Read the model definition and answer for the solid it produces. Units are mm, in the model's axes. A direction names the side the tool comes from. Round coordinates to 2 decimals unless told otherwise and drop trailing zeros. Order: outer loops, then holes, each group sorted by start corner. A loop starts at its lowest first (then second) coordinate and runs counter-clockwise, first axis right, second up. Notation, with made-up numbers: (39, 42.5) - (47, 42.5) arc R14 cw to (47, 53.5) - close; hole circle Ø7 at (32, 46). An arc over 180 degrees is marked (long way). Put each result on its own line as item: value. Start each with the question number.
Q1. Section A-A on x = 0 is taken. Give the vertices of the cut face in (y, z).
Q2. Find the intervals of material crossed by line 1 along X through (y, z) = (6, 0); line 2 along Z through (x, y) = (0, 3); line 3 along Z through (x, y) = (113.5, 9.5), in increasing order. Write a range as from..to.
Q3. Section B-B on y = 13.5 is taken. Give the vertices of the cut face in (x, z), then the cut area to 3 significant figures.
Q4. For a pull along Z with two mould halves and no side action, classify faces 1 (the face through (188.4, 4.9, 54.8)), 2 (the face through (-113.35, 5.07, -64.18)), 3 (the face through (111.43, 5.07, -66.42)) as pulls with the +Z half, pulls with the -Z half, needs draft (parallel to the pull), parting line crosses it, or undercut.
Q5. Which of the six approach directions +Z, -Z, +X, -X, +Y, -Y give full straight-line access (tool end or side, diameter ignored) to faces 4 (the face through (69, 10, -3)), 5 (the face through (-80, 15, 0)), 6 (the face through (-133.6, 4.9, -111.4))?
Q6. Section D-D on x = 65 is taken. Give the vertices of the cut face in (y, z), then the cut area to 3 significant figures.
Q7. Each of these flat-tipped pins is pushed along its axis until it touches: pin 1 Ø5 at (x, y) = (163, 7.5) entering from +Z; pin 2 Ø8 at (y, z) = (6.5, 102) entering from +X; pin 3 Ø5 at (x, y) = (155, 7.5) entering from -Z. Where does it stop, or does it pass through?
Q8. Section C-C on z = -107.5 is taken. Give the vertices of the cut face in (x, y).
from build123d import *

# Parameters (mm, degrees)
SKETCH2_R           = 120
SKETCH2_R_2         = 60
BOSS_EXTRUDE1_DEPTH = 10
BOSS_EXTRUDE2_DEPTH = 10
CIRPATTERN1_COUNT   = 3
FILLET1_R           = 80
BOSS_EXTRUDE3_DEPTH = 10


with BuildPart() as part:
    # Sketch2 → Boss-Extrude1 (new body)
    with BuildSketch(Plane(origin=(0, 0, 0), x_dir=(1, 0, 0), z_dir=(0, 1, 0))):
        with Locations(Location((0, 0, 0), (0, 0, 270))):
            Circle(SKETCH2_R)
        with Locations(Location((0, 0, 0), (0, 0, 270))):
            Circle(SKETCH2_R_2, mode=Mode.SUBTRACT)
    extrude(amount=BOSS_EXTRUDE1_DEPTH)

    # Sketch2_3 → Boss-Extrude2 (add)
    with BuildSketch(Plane(origin=(0, 0, 0), x_dir=(1, 0, 0), z_dir=(0, 1, 0))):
        with BuildLine():
            Line((183.198176877, 60), (103.923048454, 60))
            ThreePointArc((103.923048454, 60), (115.911099155, 31.058285412), (120, 0))
            ThreePointArc((120, 0), (115.911099155, -31.058285412), (103.923048454, -60))
            Line((103.923048454, -60), (183.198176877, -60))
            Line((183.198176877, -60), (193.804778595, -49.393398282))
            ThreePointArc((193.804778595, -49.393398282), (200, 0), (193.804778595, 49.393398282))
            Line((193.804778595, 49.393398282), (183.198176877, 60))
        make_face()
    boss_extrude2 = extrude(amount=BOSS_EXTRUDE2_DEPTH)

    # CirPattern1: Boss-Extrude2 ×3 about axis
    cirpattern1_axis = Axis((0, 0, 0), (0, 1, 0))
    for i in range(1, CIRPATTERN1_COUNT):
        add(boss_extrude2.rotate(cirpattern1_axis, i * 360 / CIRPATTERN1_COUNT))

    # Fillet1
    fillet1_edges = [part.edges().sort_by_distance(p)[0] for p in [
        (103.923048454, 5, -60),
        (103.923048454, 5, 60),
        (-103.923048454, 5, -60),
        (0, 5, -120),
        (0, 5, 120),
        (-103.923048454, 5, 60),
    ]]
    fillet(fillet1_edges, radius=FILLET1_R)

    # Sketch3 → Boss-Extrude3 (add)
    with BuildSketch(Plane(origin=(0, 10, 0), x_dir=(1, 0, 0), z_dir=(0, 1, 0))):
        with BuildLine():
            Line((-5.773502692, 10), (-8.660254038, 5))
            ThreePointArc((-8.660254038, 5), (-5, 8.660254038), (0, 10))
            Line((0, 10), (-5.773502692, 10))
        make_face()
        with BuildLine():
            ThreePointArc((8.660254038, 5), (10, 0), (8.660254038, -5))
            Line((8.660254038, -5), (11.547005384, 0))
            Line((11.547005384, 0), (8.660254038, 5))
        make_face()
        with BuildLine():
            Line((-5.773502692, -10), (0, -10))
            ThreePointArc((0, -10), (-5, -8.660254038), (-8.660254038, -5))
            Line((-8.660254038, -5), (-5.773502692, -10))
        make_face()
        with BuildLine():
            ThreePointArc((-8.660254038, -5), (-5, -8.660254038), (0, -10))
            ThreePointArc((0, -10), (5, -8.660254038), (8.660254038, -5))
            ThreePointArc((8.660254038, -5), (10, 0), (8.660254038, 5))
            ThreePointArc((8.660254038, 5), (5, 8.660254038), (0, 10))
            ThreePointArc((0, 10), (-5, 8.660254038), (-8.660254038, 5))
            ThreePointArc((-8.660254038, 5), (-10, 0), (-8.660254038, -5))
        make_face()
        with BuildLine():
            Line((8.660254038, 5), (11.547005384, 0))
            Line((11.547005384, 0), (22.802389662, 19.494897428))
            ThreePointArc((22.802389662, 19.494897428), (15, 25.980762114), (5.481881586, 29.494897428))
            Line((5.481881586, 29.494897428), (-5.773502692, 10))
            Line((-5.773502692, 10), (0, 10))
            ThreePointArc((0, 10), (5, 8.660254038), (8.660254038, 5))
        make_face()
        with BuildLine():
            ThreePointArc((8.660254038, -5), (5, -8.660254038), (0, -10))
            Line((0, -10), (-5.773502692, -10))
            Line((-5.773502692, -10), (5.481881586, -29.494897428))
            ThreePointArc((5.481881586, -29.494897428), (15, -25.980762114), (22.802389662, -19.494897428))
            Line((22.802389662, -19.494897428), (11.547005384, 0))
            Line((11.547005384, 0), (8.660254038, -5))
        make_face()
        with BuildLine():
            Line((-28.284271247, -10), (-5.773502692, -10))
            Line((-5.773502692, -10), (-8.660254038, -5))
            ThreePointArc((-8.660254038, -5), (-10, 0), (-8.660254038, 5))
            Line((-8.660254038, 5), (-5.773502692, 10))
            Line((-5.773502692, 10), (-28.284271247, 10))
            ThreePointArc((-28.284271247, 10), (-30, 0), (-28.284271247, -10))
        make_face()
        with BuildLine():
            ThreePointArc((5.481881586, 29.494897428), (-15, 25.980762114), (-28.284271247, 10))
            Line((-28.284271247, 10), (-5.773502692, 10))
            Line((-5.773502692, 10), (5.481881586, 29.494897428))
        make_face()
        with BuildLine():
            Line((22.802389662, 19.494897428), (11.547005384, 0))
            Line((11.547005384, 0), (22.802389662, -19.494897428))
            ThreePointArc((22.802389662, -19.494897428), (28.143131399, -10.390580113), (30, 0))
            ThreePointArc((30, 0), (28.143131399, 10.390580113), (22.802389662, 19.494897428))
        make_face()
        with BuildLine():
            Line((5.481881586, -29.494897428), (-5.773502692, -10))
            Line((-5.773502692, -10), (-28.284271247, -10))
            ThreePointArc((-28.284271247, -10), (-15, -25.980762114), (5.481881586, -29.494897428))
        make_face()
        with BuildLine():
            Line((-59.160797831, -10), (-28.284271247, -10))
            ThreePointArc((-28.284271247, -10), (-30, 0), (-28.284271247, 10))
            Line((-28.284271247, 10), (-59.160797831, 10))
            ThreePointArc((-59.160797831, 10), (-60, 0), (-59.160797831, -10))
        make_face()
        with BuildLine():
            ThreePointArc((5.481881586, 29.494897428), (15, 25.980762114), (22.802389662, 19.494897428))
            Line((22.802389662, 19.494897428), (38.240652953, 46.23475383))
            ThreePointArc((38.240652953, 46.23475383), (30, 51.961524227), (20.920144878, 56.23475383))
            Line((20.920144878, 56.23475383), (5.481881586, 29.494897428))
        make_face()
        with BuildLine():
            ThreePointArc((22.802389662, -19.494897428), (15, -25.980762114), (5.481881586, -29.494897428))
            Line((5.481881586, -29.494897428), (20.920144878, -56.23475383))
            ThreePointArc((20.920144878, -56.23475383), (30, -51.961524227), (38.240652953, -46.23475383))
            Line((38.240652953, -46.23475383), (22.802389662, -19.494897428))
        make_face()
        with BuildLine():
            ThreePointArc((38.240652953, -46.23475383), (30, -51.961524227), (20.920144878, -56.23475383))
            Line((20.920144878, -56.23475383), (26.339745962, -65.621778265))
            ThreePointArc((26.339745962, -65.621778265), (40, -69.282032303), (43.660254038, -55.621778265))
            Line((43.660254038, -55.621778265), (38.240652953, -46.23475383))
        make_face()
        with BuildLine():
            ThreePointArc((20.920144878, 56.23475383), (30, 51.961524227), (38.240652953, 46.23475383))
            Line((38.240652953, 46.23475383), (43.660254038, 55.621778265))
            ThreePointArc((43.660254038, 55.621778265), (40, 69.282032303), (26.339745962, 65.621778265))
            Line((26.339745962, 65.621778265), (20.920144878, 56.23475383))
        make_face()
        with BuildLine():
            Line((-70, -10), (-59.160797831, -10))
            ThreePointArc((-59.160797831, -10), (-60, 0), (-59.160797831, 10))
            Line((-59.160797831, 10), (-70, 10))
            ThreePointArc((-70, 10), (-80, 0), (-70, -10))
        make_face()
    extrude(amount=BOSS_EXTRUDE3_DEPTH)


solid = part.part
Findings:
1. outline: (0, -131.11) - (10, -131.11) - (10, -60) - (0, -60) - close; (0, 60) - (10, 60) - (10, 131.11) - (0, 131.11) - close; (10, -30) - (20, -30) - (20, 30) - (10, 30) - close
2. line 1: -120..-60, 60..200
2. line 2: -131.11..-60, 60..131.11
2. line 3: -65.57..65.57
3. outline: (-70, -10) - (-28.28, -10) arc R30 ccw to (5.48, -29.49) - (26.34, -65.62) arc R10 ccw to (43.66, -55.62) - (22.8, -19.49) arc R30 ccw to (22.8, 19.49) - (43.66, 55.62) arc R10 ccw to (26.34, 65.62) - (5.48, 29.49) arc R30 ccw to (-28.28, 10) - (-70, 10) arc R10 ccw to start
3. area: 5,730 mm2
4. face 1: pulls with the +Z half
4. face 2: undercut
4. face 3: pulls with the -Z half
5. face 4: +Y
5. face 5: -X, +Y
5. face 6: -X, +Y, -Y
6. outline: (0, -100.87) - (10, -100.87) - (10, 100.87) - (0, 100.87) - close
6. area: 2,020 mm2
7. pin 1: z = 60
7. pin 2: x = 69.25
7. pin 3: z = -60
8. outline: (-131.35, 0) - (53.33, 0) - (53.33, 10) - (-131.35, 10) - close
